from build123d import *

# Parameters (mm, degrees)
SKETCH1_W           = 60
SKETCH1_H           = 70
BOSS_EXTRUDE1_DEPTH = 100
SKETCH2_W           = 10
SKETCH2_H           = 40
BOSS_EXTRUDE2_DEPTH = 10
SKETCH5_W           = 60
SKETCH5_H           = 5
BOSS_EXTRUDE4_DEPTH = 10
SKETCH6_R           = 1.5
CUT_EXTRUDE4_DEPTH  = 10
SKETCH7_W           = 60
SKETCH7_H           = 30
CUT_EXTRUDE5_DEPTH  = 10


with BuildPart() as part:
    # Sketch1 → Boss-Extrude1 (new body)
    with BuildSketch(Plane(origin=(0, 0, 0), x_dir=(1, 0, 0), z_dir=(0, 1, 0))):
        with Locations((30, 35)):
            Rectangle(SKETCH1_W, SKETCH1_H)
    extrude(amount=BOSS_EXTRUDE1_DEPTH)

    # Sketch2 → Boss-Extrude2 (add)
    with BuildSketch(Plane(origin=(0, 100, 0), x_dir=(1, 0, 0), z_dir=(0, 1, 0))):
        with Locations((55, 35)):
            Rectangle(SKETCH2_W, SKETCH2_H)
    extrude(amount=BOSS_EXTRUDE2_DEPTH)

    # Sketch5 → Boss-Extrude4 (add)
    with BuildSketch(Plane(origin=(0, 100, 0), x_dir=(1, 0, 0), z_dir=(0, 1, 0))):
        with Locations((30, 67.5)):
            Rectangle(SKETCH5_W, SKETCH5_H)
    extrude(amount=BOSS_EXTRUDE4_DEPTH)

    # Sketch6 → Cut-Extrude4 (cut)
    with BuildSketch(Plane(origin=(0, 0, -70), x_dir=(-1, 0, 0), z_dir=(0, 0, -1))):
        with Locations((-50, 105)):
            Circle(SKETCH6_R)
        with Locations((-10, 105)):
            Circle(SKETCH6_R)
    extrude(amount=-CUT_EXTRUDE4_DEPTH, mode=Mode.SUBTRACT)

    # Sketch7 → Cut-Extrude5 (cut)
    with BuildSketch(Plane.XZ):
        with Locations((30, -55)):
            Rectangle(SKETCH7_W, SKETCH7_H)
    extrude(amount=-CUT_EXTRUDE5_DEPTH, mode=Mode.SUBTRACT)


solid = part.part
Here's how the part is built. I have some questions about the finished solid (model axes, mm). A direction names the side the tool comes from. Coordinates: 2 decimals unless noted, no trailing zeros. Order: outer loops, then holes, each group sorted by start corner. A loop starts at its lowest first (then second) coordinate and runs counter-clockwise, first axis right, second up. Notation, with made-up numbers: (-10.75, 83) -> (46.25, 83) arc R12 cw to (46.25, 89) -> close; hole circle Ø8 at (88, 11.25). An arc over 180 degrees is marked (long way). Answer in a Markdown table with one row per item.
(1) I want a section at C-C on z = -21. List the corners of the cut face in (x, y) for me.
Answer key:
| item | result |
|---|---|
| outline | (0, 0) -> (60, 0) -> (60, 110) -> (50, 110) -> (50, 100) -> (0, 100) -> close |
(2) Thinking about a two-plate mould opening in Y: for faces 6 (the face through (10.195, 106.487, -67.535)), 7 (the face through (55, 105, -55)), 8 (the face through (30, 0, -20)), which applies, +Y half, -Y half, draft (parallel to the pull), parting line (faces both ways), or undercut?
Answer key:
| item | result |
|---|---|
| face 6 | undercut |
| face 7 | draft |
| face 8 | -Y half |
(3) On a 3-axis mill with a long thin cutter (end or side, diameter ignored), from which of +Z, -Z, +X, -X, +Y, -Y can I reach the whole of each face in a straight line? I mean faces 1 (the face through (30, 10, -55)), 2 (the face through (50, 105, -35)), 3 (the face through (55, 105, -15)), 4 (the face through (50.195, 106.487, -67.535)), 5 (the face through (30, 105, -65)). Say none if no direction works.
Answer key:
| item | result |
|---|---|
| face 1 | -Z, +X, -X, -Y |
| face 2 | +Z, -X, +Y |
| face 3 | +Z, +X, -X, +Y |
| face 4 | -Z |
| face 5 | +X, -X, +Y |
(4) I want a section at D-D on x = 45. List the corners of the cut face in (y, z) for me, then the cut area to 3 significant figures.
Answer key:
| item | result |
|---|---|
| outline | (0, -40) -> (10, -40) -> (10, -70) -> (110, -70) -> (110, -65) -> (100, -65) -> (100, 0) -> (0, 0) -> close |
| area | 6,750 mm^2 |
(5) Will these pins go through, and if not, where does the flat tip stop? pin 1 Ø8 at (x, y) = (23, 3.5) entering from -Z; pin 2 Ø15 at (x, z) = (24.5, -50) entering from -Y; pin 3 Ø1.8 at (x, y) = (50, 105) entering from +Z.
Answer key:
| item | result |
|---|---|
| pin 1 | z = -40 |
| pin 2 | y = 10 |
| pin 3 | z = -15 |
(6) Please list where these lines run through material, in increasing order: probe 1 along X at (y, z) = (105, -66); probe 2 along Y at (x, z) = (50, -67.85); probe 3 along Y at (x, z) = (26, -53).
Answer key:
| item | result |
|---|---|
| probe 1 | 0 to 8.5, 11.5 to 48.5, 51.5 to 60 |
| probe 2 | 10 to 103.5, 106.5 to 110 |
| probe 3 | 10 to 100 |
(7) I want a section at B-B on x = 10. List the corners of the cut face in (y, z) for me.
Answer key:
| item | result |
|---|---|
| outline | (0, -40) -> (10, -40) -> (10, -70) -> (103.5, -70) -> (103.5, -65) -> (100, -65) -> (100, 0) -> (0, 0) -> close; (106.5, -70) -> (110, -70) -> (110, -65) -> (106.5, -65) -> close |
(8) I want a section at A-A on y = 105. List the corners of the cut face in (x, z) for me, then the cut area to 3 significant figures.
Answer key:
| item | result |
|---|---|
| outline | (0, -70) -> (8.5, -70) -> (8.5, -65) -> (0, -65) -> close; (11.5, -70) -> (48.5, -70) -> (48.5, -65) -> (11.5, -65) -> close; (50, -55) -> (60, -55) -> (60, -15) -> (50, -15) -> close; (51.5, -70) -> (60, -70) -> (60, -65) -> (51.5, -65) -> close |
| area | 670 mm^2 |
